For this review, take the finished solid that the model builds, in its own axes (mm). A direction names the side the tool comes from. Give positions to 0.01 mm unless a question says otherwise; leave off trailing zeros. Write each loop counter-clockwise with the first axis right and the second up, starting at its lowest first coordinate (ties: lowest second). Pieces come first, ordered by that corner, then holes.
from build123d import *

# Parameters (mm, degrees)
SKETCH_1_R          = 2.5
EXTRUDE_1_DEPTH     = 5
SKETCH_2_R          = 1.5
CUT_EXTRUDE_1_DEPTH = 15
SKETCH_3_R          = 1.5
EXTRUDE_4_DEPTH     = 1.5


with BuildPart() as part:
    # 草图1 → 凸台-拉伸1 (new, symmetric)
    with BuildSketch(Plane(origin=(0, 0, 0), x_dir=(0, 0, -1), z_dir=(1, 0, 0))):
        Circle(SKETCH_1_R)
    extrude(amount=EXTRUDE_1_DEPTH, both=True)

    # 草图2 → 切除-拉伸1 (cut)
    with BuildSketch(Plane(origin=(0, 0, 0), x_dir=(0, 0, -1), z_dir=(1, 0, 0))):
        Circle(SKETCH_2_R)
    extrude(amount=-CUT_EXTRUDE_1_DEPTH, mode=Mode.SUBTRACT)

    # 草图3 → 凸台-拉伸4 (add, symmetric)
    with BuildSketch(Plane(origin=(5, 0, 0), x_dir=(0, 0, -1), z_dir=(1, 0, 0))):
        Circle(SKETCH_3_R)
    extrude(amount=EXTRUDE_4_DEPTH, both=True)


solid = part.part
(1) Tool access review of faces 4 (the cylindrical face through (-2.46, 0.07, 1.5)), 5 (the flat face through (5, -2, 0)), 6 (the flat face through (-5, -2, 0)): name each direction out of +Z, -Z, +X, -X, +Y, -Y from which nothing blocks a thin tool from reaching the whole face with its end or side.
(2) We need section B-B (x = -1). Write out the cut boundary in (y, z), and give its area (3 significant figures).
(3) We need section A-A (z = 0). Write out the cut boundary in (x, y), and give its area (3 significant figures).
(4) The part is to be moulded in two halves that separate along Z. For faces 1 (the flat face through (6.5, 0, 0)), 2 (the cylindrical face through (5.76, 0.07, 1.5)), 3 (the flat face through (0, 0, 0)), say which applies: +Z half, -Z half, draft (parallel to the pull), parting line (faces both ways), or undercut.
(5) We need section D-D (x = 1). Write out the cut boundary in (y, z).
(6) Clearance check with a flat-ended pin moving along its axis: pin 1 Ø1.5 at (x, z) = (3, 0.5) entering from -Y. State where the tip first meets the part, or that it passes through.
(7) For L1, parallel to Y at x = -3.95, z = 0; L2, parallel to Y at x = -2, z = -1.25; L3, parallel to X at y = 2, z = 0.25, list the stretches that pass through material, from the lowest coordinate up.
The answers:
1. face 4: -X
1. face 5: +X
1. face 6: +Z, -Z, -X, +Y, -Y
2. outline: circle Ø5 at (0, 0); hole circle Ø3 at (0, 0)
2. area: 12.6 mm2
3. outline: (-5, -2.5) - (5, -2.5) - (5, -1.5) - (6.5, -1.5) - (6.5, 1.5) - (5, 1.5) - (5, 2.5) - (-5, 2.5) - (-5, 1.5) - (0, 1.5) - (0, -1.5) - (-5, -1.5) - close
3. area: 39.5 mm2
4. face 1: draft
4. face 2: parting line
4. face 3: undercut
5. outline: circle Ø5 at (0, 0)
6. pin 1: stops at y = -2.5
7. L1: y = -2.5 to -1.5, 1.5 to 2.5
7. L2: y = -2.17 to -0.83, 0.83 to 2.17
7. L3: x = -5 to 5
